Autodesk Inventor part; units mm, degrees
ref_plane "YZ Plane" through (0, 0, 0) normal (1, 0, 0) x (0, 1, 0)
ref_plane "XZ Plane" through (0, 0, 0) normal (0, 1, 0) x (-1, 0, 0)
ref_plane "XY Plane" through (0, 0, 0) normal (0, 0, 1) x (1, 0, 0)
sketch "Sketch1" plane through (0, 0, 0) normal (0, 1, 0) x (-1, 0, 0)
  line L0 (0, -14) -> (0, 14)
  line L1 (-14, 0) -> (14, 0)
  line L2 (14, 0) -> (-14, 0)
  line L3 (0, -14) -> (0, 14)
  line L4 (2.5943, 3.655) -> (-2.5943, 3.655)
  line L5 (-3.655, 2.5943) -> (-3.655, -2.5943)
  line L6 (-2.5943, -3.655) -> (2.5943, -3.655)
  line L7 (3.655, -2.5943) -> (3.655, 2.5943)
  line L8 (-3.655, 3.655) -> (3.655, -3.655) construction
  line L9 (10, 10) -> (10, 2.63)
  line L10 (10, 2.63) -> (8.5, 2.63)
  line L11 (10, 10) -> (2.63, 10)
  line L12 (2.63, 10) -> (2.63, 8.5)
  line L13 (-10, 10) -> (-2.63, 10)
  line L14 (-2.63, 10) -> (-2.63, 8.5)
  line L15 (-10, 8.5) -> (-10, 10)
  line L16 (-10, 10) -> (-8.5, 10)
  line L17 (-8.5, 2.63) -> (-10, 2.63)
  line L18 (-10, 2.63) -> (-10, 10)
  line L19 (-10, -10) -> (-8.5, -10)
  line L20 (-8.5, -2.63) -> (-10, -2.63)
  line L21 (-10, -2.63) -> (-10, -10)
  line L22 (-10, -10) -> (-2.63, -10)
  line L23 (-2.63, -10) -> (-2.63, -8.5)
  line L24 (-10, -8.5) -> (-10, -10)
  line L25 (10, -10) -> (8.5, -10)
  line L26 (8.5, -2.63) -> (10, -2.63)
  line L27 (10, -2.63) -> (10, -10)
  line L28 (10, -10) -> (2.63, -10)
  line L29 (2.63, -10) -> (2.63, -8.5)
  line L30 (10, -8.5) -> (10, -10)
  circle A0 centre (0, 0) radius 2.095
  line L31 (5.995, -10) -> (2.63, -10)
  line L32 (-2.63, -10) -> (-5.995, -10)
  line L33 (10, -10) -> (2.63, -10)
  line L34 (-2.63, -10) -> (-10, -10)
  line L35 (10, -5.995) -> (10, -2.63)
  line L36 (10, 2.63) -> (10, 5.995)
  line L37 (10, 10) -> (10, 2.63)
  line L38 (10, -2.63) -> (10, -10)
  line L39 (-5.995, 10) -> (-2.63, 10)
  line L40 (2.63, 10) -> (5.995, 10)
  line L41 (-10, 10) -> (-2.63, 10)
  line L42 (2.63, 10) -> (10, 10)
  line L43 (-10, 5.995) -> (-10, 2.63)
  line L44 (-10, -2.63) -> (-10, -5.995)
  line L45 (-10, -10) -> (-10, -2.63)
  line L46 (-10, 2.63) -> (-10, 10)
  line L47 (-2.63, -8.5) -> (-5.995, -8.5)
  line L48 (-8.5, -5.995) -> (-8.5, -2.63)
  line L49 (-8.5, -5.995) -> (-7.0557, -5.995)
  line L50 (-5.995, -8.5) -> (-5.995, -7.0557)
  line L51 (-5.995, 7.0557) -> (-5.995, 8.5)
  line L52 (2.63, 8.5) -> (5.995, 8.5)
  line L53 (8.5, 2.63) -> (8.5, 5.995)
  line L54 (8.5, 5.995) -> (7.0557, 5.995)
  line L55 (5.995, 8.5) -> (5.995, 7.0557)
  line L56 (2.63, -8.5) -> (5.995, -8.5)
  line L57 (9.5607, -8.5) -> (10, -8.5)
  line L58 (8.5, -10) -> (8.5, -9.5607)
  line L59 (8.5, -5.995) -> (8.5, -2.63)
  line L60 (7.0557, -5.995) -> (8.5, -5.995)
  line L61 (5.995, -7.0557) -> (5.995, -8.5)
  line L62 (3.655, 3.655) -> (-0.5303, -0.5303) construction
  line L63 (-1.4814, -1.4814) -> (-3.655, -3.655) construction
  line L64 (-8.5, 10) -> (-8.5, 9.5607)
  line L65 (-8.5, 5.995) -> (-8.5, 2.63)
  line L66 (-2.63, 8.5) -> (-5.995, 8.5)
  line L67 (-9.5607, 8.5) -> (-10, 8.5)
  line L68 (-7.0557, 5.995) -> (-8.5, 5.995)
  line L69 (-3.655, 2.5943) -> (-7.0557, 5.995)
  line L70 (-2.5943, 3.655) -> (-5.995, 7.0557)
  line L71 (5.995, 7.0557) -> (2.5943, 3.655)
  line L72 (7.0557, 5.995) -> (3.655, 2.5943)
  line L73 (7.0557, -5.995) -> (3.655, -2.5943)
  line L74 (5.995, -7.0557) -> (2.5943, -3.655)
  line L75 (-2.5943, -3.655) -> (-5.995, -7.0557)
  line L76 (-3.655, -2.5943) -> (-7.0557, -5.995)
  dimension "d26" = 4.19
  dimension "d0" = 20
  dimension "d1" = 20
  dimension "d2" = 7.31
  dimension "d3" = 7.31
  dimension "d4" = 20
  dimension "d5" = 11.99
  dimension "d6" = 11.99
  dimension "d11" = 7.37
  dimension "d12" = 1.5
  dimension "d13" = 7.37
  dimension "d14" = 1.5
  dimension "d15" = 7.37
  dimension "d16" = 1.5
  dimension "d17" = 7.37
  dimension "d18" = 1.5
  dimension "d19" = 7.37
  dimension "d20" = 7.37
  dimension "d21" = 1.5
  dimension "d22" = 1.5
  dimension "d23" = 7.37
  dimension "d24" = 7.37
  dimension "d25" = 1.5
extrude "Extrusion1" add sketch "Sketch1" along normal blind 200 contours L6 L75 L50 L47 L23 L22 L19 L21 L20 L48 L49 L76 L5 L1 A0 L0 | L0 A0 L1 L7 L73 L60 L59 L26 L27 L25 L28 L29 L56 L61 L74 L6 | L1 L5 L69 L68 L65 L17 L18 L15 L13 L14 L66 L51 L70 L4 L0 A0 | A0 L0 L4 L71 L55 L52 L12 L11 L9 L10 L53 L54 L72 L7 L1
fillet "Fillet1" radius 0.5 20 edges at (10, 100, 10) (2.63, 100, 10) (-2.63, 100, 10) (-2.63, 100, 8.5) (10, 100, 2.63) (8.5, 100, 2.63) (10, 100, -2.63) (8.5, 100, -2.63) (10, 100, -10) (2.63, 100, -8.5) (-2.63, 100, -10) (-2.63, 100, -8.5) (2.63, 100, -10) (-10, 100, -10) (-8.5, 100, -2.63) (-10, 100, -2.63) (-8.5, 100, 2.63) (-10, 100, 2.63) (-10, 100, 10) (2.63, 100, 8.5)
fillet "Fillet2" radius 0.75 24 edges at (-7.0557, 100, 5.995) (-3.655, 100, 2.5943) (-8.5, 100, -5.995) (-7.0557, 100, -5.995) (-5.995, 100, -8.5) (3.655, 100, -2.5943) (7.0557, 100, -5.995) (-2.5943, 100, 3.655) (-5.995, 100, 7.0557) (3.655, 100, 2.5943) (7.0557, 100, 5.995) (8.5, 100, 5.995) (8.5, 100, -5.995) (2.5943, 100, 3.655) (5.995, 100, 7.0557) (5.995, 100, 8.5) (-5.995, 100, 8.5) (-8.5, 100, 5.995) (2.5943, 100, -3.655) (5.995, 100, -7.0557) (5.995, 100, -8.5) (-5.995, 100, -7.0557) (-2.5943, 100, -3.655) (-3.655, 100, -2.5943)
properties part number "Profile_Len_160mm"
Check sheet for the modelled part. Datum: model origin and axes. Units: mm. A direction names the side the tool comes from. Round coordinates to 2 decimals unless told otherwise and drop trailing zeros. Write each loop counter-clockwise with the first axis right and the second up, starting at its lowest first coordinate (ties: lowest second). Pieces come first, ordered by that corner, then holes. Notation, with made-up numbers: M 85.5,29 L 91.5,29 A38 ccw 91.5,67 Z; hole C 27,66.5 d2. An arc over 180 degrees is marked long. Write item = value, one per line. Start each with the question number.
1. Gauge pin test, flat ends, axial feed: pin 1 (5 mm diameter, centred on x = 0, y = 58.5, fed in from +Z); pin 2 (1.4 mm diameter, centred on y = 80, z = -0.5, fed in from +X) (3 decimals); pin 3 (1 mm diameter, centred on y = 154, z = -0.5, fed in from -X) (3 decimals). Record the tip position at first contact, or that the pin passes through.
2. Section check A-A, the plane z = 0. Record the cut outline in (x, y) (3 decimals).
3. Scan lines: line 1 (X direction, y = 83, z = 0) (3 decimals); line 2 (X direction, y = 125, z = 8.25); line 3 (Z direction, x = -7.75, y = 147) (3 decimals). Record each from-to range of solid material in increasing order. Write a range as [from, to].
4. Tool access check on faces 4 (the flat face through (0, 99, 3.655)), 5 (the flat face through (0, 99, -3.655)), 6 (the flat face through (-3.655, 99, 0)). Record the directions out of +Z, -Z, +X, -X, +Y, -Y that give a thin tool (end or side, any length) a straight path to the whole face; none if there is none.
5. Release check for a two-part mould opening along Z. For faces 1 (the flat face through (3.655, 99, 0)), 2 (the flat face through (-10, 99, 6)), 3 (the flat face through (-6, 99, -10)) record: pulls with the +Z half, pulls with the -Z half, needs draft (parallel to the pull), parting line crosses it, or undercut.
6. Section check B-B, the plane x = 0. Record the cut outline in (y, z) (3 decimals).
Results found:
q1.pin_1 = 3.69
q1.pin_2 = 3.655
q1.pin_3 = -3.655
q2.outline = M -3.655,0 L -2.095,0 L -2.095,200 L -3.655,200 Z; M 2.095,0 L 3.655,0 L 3.655,200 L 2.095,200 Z
q3.line_1 = [-3.655, -2.095], [2.095, 3.655]
q3.line_2 = [-10, -5.8], [5.8, 10]
q3.line_3 = [-10, -5.995], [5.995, 10]
q4.face_4 = +Z, +Y, -Y
q4.face_5 = -Z, +Y, -Y
q4.face_6 = -X, +Y, -Y
q5.face_1 = undercut
q5.face_2 = needs draft
q5.face_3 = pulls with the -Z half
q6.outline = M 0,-3.655 L 200,-3.655 L 200,-2.095 L 0,-2.095 Z; M 0,2.095 L 200,2.095 L 200,3.655 L 0,3.655 Z
